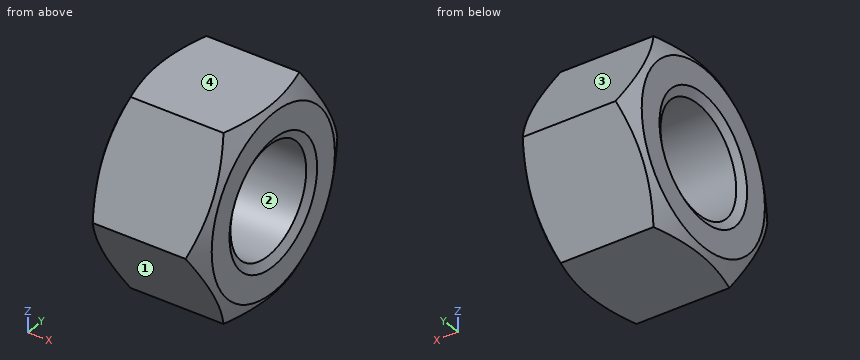
Autodesk Inventor part; units mm, degrees
ref_plane "Work Plane1" through (-25.1166, 0, 0) normal (0, -0.866, -0.5) x (1, 0, 0)
ref_plane "YZ Plane" through (0, 0, 0) normal (1, 0, 0) x (0, 1, 0)
ref_plane "XZ Plane" through (0, 0, 0) normal (0, 1, 0) x (-1, 0, 0)
sketch "Эскиз1" plane through (0, 0, 0) normal (1, 0, 0) x (0, 1, 0)
  line L0 (-13.8564, 0) -> (-6.9282, 12)
  line L1 (-6.9282, 12) -> (6.9282, 12)
  line L2 (6.9282, 12) -> (13.8564, 0)
  line L3 (13.8564, 0) -> (6.9282, -12)
  line L4 (6.9282, -12) -> (-6.9282, -12)
  line L5 (-6.9282, -12) -> (-13.8564, 0)
  point P0 (0, 0)
  point P1 (0, 0)
  dimension "d0" = 27.7128
extrude "Базовый элемент" add sketch "Эскиз1" along normal blind 14.8
sketch "Эскиз2" plane through (0, 0, 0) normal (0, 0, 1) x (1, 0, 0)
  line L0 (0, 6.9282) -> (0, 13.8564)
  line L1 (0, 13.8564) -> (14.8, 13.8564)
  line L2 (14.8, 6.9282) -> (14.8, 13.8564)
  line L3 (-2.96, 0) -> (17.76, 0)
  line L4 (1.5048, 13.8564) -> (0, 11.25)
  line L5 (13.2952, 13.8564) -> (14.8, 11.25)
  dimension "d3" = 30
  dimension "d4" = 30
  dimension "d5" = 22.5
  dimension "d6" = 22.5
revolve "Фаска1" cut sketch "Эскиз2" angle 360 about axis through (-10, 0, 0) along (1, 0, 0)
sketch "Эскиз3" plane through (14.8, 0, 0) normal (1, 0, 0) x (0, 0, -1)
  arc A0 (-0.625, -1.0825) -> (0.625, -1.0825) centre (0, 0) ccw
hole "Резьба" at (14.8, 0, 0) direction (-1, 0, 0) diameter 13.835 end through all
chamfer "Фаска2" distance 1.0825 angle 30 1 edges at (14.8, 0, 6.9175) measured on face at (14.8, 9.6801, -1.1754)
chamfer "Фаска3" distance 1.0825 angle 30 1 edges at (0, 0, 6.9175) measured on face at (0, 9.6801, -1.1754)
ref_plane "Work Plane1" through (-25.1166, 0, 0) normal (0, -0.866, -0.5) x (1, 0, 0)
equation "\"d0\" = 1.1547 * SW"
equation "\"d1\" = KOH"
equation "\"d3\" = ANG1"
equation "\"d4\" = ANG2"
equation "\"d5\" = SW0"
equation "\"d6\" = SW01"
equation "\"d8\" = -0.5 * GD1 + 0.5 * NND"
equation "\"d40\" = -0.5 * GD1 + 0.5 * NND"
equation "\"d10\" = -0.5 * GD1 + 0.5 * NND"
equation "\"d41\" = -0.5 * GD1 + 0.5 * NND"
equation "\"ANG1\" = 30deg"
equation "\"ANG2\" = 30deg"
equation "\"NND\" = 16"
equation "\"KOH\" = 14.8"
equation "\"SW\" = 24"
equation "\"SW0\" = 22.5"
equation "\"SW01\" = SW0"
equation "\"GUL\" = 0.541266 * PTC"
equation "\"LADI\" = 22.8"
equation "\"TOA\" = 30deg"
equation "\"FAWI\" = 30deg"
equation "\"PTC\" = 2"
equation "\"THREADDIA\" = 16"
equation "\"E0\" = 1.155 * SW"
equation "\"GAL\" = 0.541266 * PTC"
properties part number "M16-6H ГОСТ ISO 4032-2014" material "Сталь, мягкая"
Could you check a few things on this model? Use its own coordinates, in mm. Face numbers are marked on the shaded views. Round coordinates to 2 decimals unless told otherwise and drop trailing zeros. Write each loop counter-clockwise with the first axis right and the second up, starting at its lowest first coordinate (ties: lowest second). Pieces come first, ordered by that corner, then holes. Notation, with made-up numbers: (12.25, -26.75) - (42.25, -26.75) arc R31 cw to (42.25, 5.25) - close; hole circle Ø1 at (-11.5, 71.5). An arc over 180 degrees is marked (long way). Put each result on its own line as item: value. Start each with the question number.
(1) I want a section at A-A, the plane y = 0. Please give me the cut outline in (x, z).
(2) I want a section at B-B, the plane x = 6.5. Please give me the cut outline in (y, z) (1 decimal).
(3) Thinking about a two-plate mould opening in Y: for the marked faces 1, 2, 3 and 4, which applies, released by +Y, released by -Y, zero draft, split by the parting line, or undercut?
(4) Will these pins go through, and if not, where does the flat tip stop? pin 1 (11 mm diameter, centred on y = 0, z = 0, fed in from +X); pin 2 (5 mm diameter, centred on x = 9.5, z = 1.5, fed in from +Y).
(5) I need wall thicknesses on probe 1 along Z at (x, y) = (5.5, 0); probe 2 along Y at (x, z) = (10.5, -3.25); probe 3 along Y at (x, z) = (10, 2.25). Which ranges of each line are inside material? Lowest first, please.
Here are the results:
1. outline: (0, -11.25) - (0.43, -12) - (14.37, -12) - (14.8, -11.25) - (14.8, -8) - (14.18, -6.92) - (0.62, -6.92) - (0, -8) - close; (0, 8) - (0.62, 6.92) - (14.18, 6.92) - (14.8, 8) - (14.8, 11.25) - (14.37, 12) - (0.43, 12) - (0, 11.25) - close
2. outline: (-13.9, 0) - (-6.9, -12) - (6.9, -12) - (13.9, 0) - (6.9, 12) - (-6.9, 12) - close; hole circle Ø13.8 at (0, 0)
3. face 1: released by -Y
3. face 2: undercut
3. face 3: released by +Y
3. face 4: zero draft
4. pin 1: passes through
4. pin 2: stops at y = 13.86
5. probe 1: z = -12 to -6.92, 6.92 to 12
5. probe 2: y = -11.98 to -6.11, 6.11 to 11.98
5. probe 3: y = -12.56 to -6.54, 6.54 to 12.56
